Here's how the part is built. I have some questions about the finished solid (model axes, mm). A direction names the side the tool comes from. Give positions to 0.01 mm unless a question says otherwise; leave off trailing zeros. Write each loop counter-clockwise with the first axis right and the second up, starting at its lowest first coordinate (ties: lowest second). Pieces come first, ordered by that corner, then holes. Notation, with made-up numbers: (22.5, 14.5) -> (57.5, 14.5) arc R18 cw to (57.5, 42.5) -> close; hole circle Ø10 at (3.5, 0.5). An arc over 180 degrees is marked (long way). Use CSV: the item, a comma, the result in double quotes. Start each with the question number.
(1) Suppose I cut it at C-C on z = -9.5. List the corners of the cut face in (x, y) for me, plus the area to 3 significant figures.
(2) For pin 1 Ø6 at (x, y) = (-27.5, -1) entering from -Z; pin 2 Ø6 at (x, y) = (64, 7) entering from +Z; pin 3 Ø10 at (x, z) = (76.5, -4.5) entering from -Y, each with a flat end and sliding along its axis, tell me the tip position at first contact or that it passes through.
(3) Suppose I cut it at D-D on x = -27.5. List the corners of the cut face in (y, z) for me.
(4) I need wall thicknesses on L1, parallel to X at y = 3.5, z = 0; L2, parallel to X at y = -7, z = 0; L3, parallel to X at y = 7.5, z = 7.5. Which ranges of each line are inside material? Lowest first, please. Write a range as [from, to].
(5) If we mould it in two halves opening along Z, with no side actions, what happens to faces 4 (the cylindrical face through (93.14, -0.17, -0.59)), 5 (the flat face through (-55.353, 0, 0)), 6 (the cylindrical face through (68.14, -0.17, -0.59)), 7 (the cylindrical face through (36.176, 11.446, -3.604))? For each: pulls with the +Z half, pulls with the -Z half, needs draft (parallel to the pull), parting line crosses it, or undercut.
(6) Suppose I cut it at B-B on y = 0. List the corners of the cut face in (x, z) for me, plus the area to 3 significant figures.
(7) Suppose I cut it at A-A on z = 0. List the corners of the cut face in (x, y) for me, plus the area to 3 significant figures.
(8) Which directions (+Z, -Z, +X, -X, +Y, -Y) give clear straight access to the entire face, cutting with the end or side of a thin tool? Please do faces 1 (the cylindrical face through (-36.604, 11.923, -3.755)), 2 (the flat face through (-38.823, -3, 5.4)), 3 (the flat face through (-34.323, 7, -10)).
from build123d import *

# Parameters (mm, degrees)
CUT_EXTRUDE1_DEPTH      = 111.105444252
CUT_EXTRUDE1_DEPTH_BACK = 111.105444252
SKETCH2_R               = 4.5


with BuildPart() as part:
    # Sketch1 → Revolve1 (revolve)
    with BuildSketch(Plane.XY):
        Polygon((108.677085229, 12), (-34.322914771, 12), (-34.322914771, 12.5), (-38.822914771, 12.5), (-38.822914771, 6), (-55.352914771, 6), (-55.352914771, 0), (108.677085229, 0), align=None)
    revolve(axis=Axis((108.677085229, 0, 0), (-1, 0, 0)))

    # Sketch2 → Cut-Extrude1 (cut, two sides: drawn at the far end of the back side and taken through both)
    with BuildSketch(Plane(origin=(0, 0, 0), x_dir=(1, 0, 0), z_dir=(0, 1, 0)).offset(-CUT_EXTRUDE1_DEPTH_BACK)):
        with Locations(Location((88.677085229, 0, 0), (0, 0, 270))):
            Circle(SKETCH2_R)
        with Locations(Location((63.677085229, 0, 0), (0, 0, 270))):
            Circle(SKETCH2_R)
    extrude(amount=CUT_EXTRUDE1_DEPTH + CUT_EXTRUDE1_DEPTH_BACK, mode=Mode.SUBTRACT)


solid = part.part
Geometry says:
1,outline,"(-38.82, -8.12) -> (-34.32, -8.12) -> (-34.32, -7.33) -> (108.68, -7.33) -> (108.68, 7.33) -> (-34.32, 7.33) -> (-34.32, 8.12) -> (-38.82, 8.12) -> close"
1,area,"2,170 mm²"
2,pin 1,"z = -12"
2,pin 2,"z = 11.31"
2,pin 3,"y = -12"
3,outline,"circle Ø24 at (0, 0)"
4,L1,"[-55.35, 59.18], [68.18, 84.18], [93.18, 108.68]"
4,L2,"[-38.82, 59.18], [68.18, 84.18], [93.18, 108.68]"
4,L3,"[-38.82, 108.68]"
5,face 4,"undercut"
5,face 5,"needs draft"
5,face 6,"undercut"
5,face 7,"parting line crosses it"
6,outline,"(-55.35, -6) -> (-38.82, -6) -> (-38.82, -12.5) -> (-34.32, -12.5) -> (-34.32, -12) -> (108.68, -12) -> (108.68, 12) -> (-34.32, 12) -> (-34.32, 12.5) -> (-38.82, 12.5) -> (-38.82, 6) -> (-55.35, 6) -> close; hole circle Ø9 at (63.68, 0); hole circle Ø9 at (88.68, 0)"
6,area,"3,620 mm²"
7,outline,"(-55.35, -6) -> (-38.82, -6) -> (-38.82, -12.5) -> (-34.32, -12.5) -> (-34.32, -12) -> (59.18, -12) -> (59.18, 12) -> (-34.32, 12) -> (-34.32, 12.5) -> (-38.82, 12.5) -> (-38.82, 6) -> (-55.35, 6) -> close; (68.18, -12) -> (84.18, -12) -> (84.18, 12) -> (68.18, 12) -> close; (93.18, -12) -> (108.68, -12) -> (108.68, 12) -> (93.18, 12) -> close"
7,area,"3,310 mm²"
8,face 1,"+X, -X"
8,face 2,"-X"
8,face 3,"+X"
